from build123d import *

# Parameters (mm, degrees)
SKETCH1_W                 = 60
SKETCH1_H                 = 50
BOSS_EXTRUDE1_DEPTH       = 6.35
CUT_EXTRUDE1_DEPTH        = 6.35
M3_5X0_6_TAPPED_HOLE1_D   = 2.9
M4X0_7_TAPPED_HOLE1_D     = 3.3
M4X0_7_TAPPED_HOLE1_DEPTH = 6.35
M4X0_7_TAPPED_HOLE1_TIP   = 0.991420021


with BuildPart() as part:
    # Sketch1 → Boss-Extrude1 (new body)
    with BuildSketch(Plane(origin=(0, 0, 0), x_dir=(1, 0, 0), z_dir=(0, 1, 0))):
        with Locations((-30, -25)):
            Rectangle(SKETCH1_W, SKETCH1_H)
    extrude(amount=BOSS_EXTRUDE1_DEPTH)

    # Sketch2 → Cut-Extrude1 (cut)
    with BuildSketch(Plane(origin=(0, 6.35, 0), x_dir=(1, 0, 0), z_dir=(0, 1, 0))):
        with BuildLine():
            Line((-26.825, -34.482582718), (-26.825, -20))
            Line((-26.825, -20), (-33.175, -20))
            Line((-33.175, -20), (-33.175, -34.482582718))
            ThreePointArc((-33.175, -34.482582718), (-30, -35), (-26.825, -34.482582718))
        make_face()
        with BuildLine():
            Line((-33.175, -20), (-26.825, -20))
            Line((-26.825, -20), (-26.825, -34.482582718))
            ThreePointArc((-26.825, -34.482582718), (-21.88365846, -30.841660723), (-20, -25))
            ThreePointArc((-20, -25), (-35.841660723, -16.88365846), (-33.175, -34.482582718))
            Line((-33.175, -34.482582718), (-33.175, -20))
        make_face()
        with BuildLine():
            Line((-26.825, -50), (-26.825, -34.482582718))
            ThreePointArc((-26.825, -34.482582718), (-30, -35), (-33.175, -34.482582718))
            Line((-33.175, -34.482582718), (-33.175, -50))
            Line((-33.175, -50), (-26.825, -50))
        make_face()
    extrude(amount=-CUT_EXTRUDE1_DEPTH, mode=Mode.SUBTRACT)

    # M3.5x0.6 Tapped Hole1 (through all)
    with Locations(Plane(origin=(-26.376533369, 6.35, 11.477038432), x_dir=(0, 0, 1), z_dir=(0, 1, 0))):
        with Locations((0, 0), (3.623466631, -13.522961568), (17.146428199, -17.146428199), (23.422456505, 6.276028306)):
            Hole(M3_5X0_6_TAPPED_HOLE1_D / 2)

    # M4x0.7 Tapped Hole1
    with Locations(Plane(origin=(-8, 3.175, 0), x_dir=(-1, 0, 0), z_dir=(0, 0, -1))):
        with Locations((0, 0), (22, 0), (44, 0)):
            Hole(M4X0_7_TAPPED_HOLE1_D / 2, depth=M4X0_7_TAPPED_HOLE1_DEPTH)
            with Locations((0, 0, -(M4X0_7_TAPPED_HOLE1_DEPTH + M4X0_7_TAPPED_HOLE1_TIP / 2))):  # 118° drill point
                Cone(0, M4X0_7_TAPPED_HOLE1_D / 2, M4X0_7_TAPPED_HOLE1_TIP, mode=Mode.SUBTRACT)


solid = part.part
Part model, mm, in its own coordinate system. A direction names the side the tool comes from. Give positions to 0.01 mm unless a question says otherwise; leave off trailing zeros. Order: outer loops, then holes, each group sorted by start corner. A loop starts at its lowest first (then second) coordinate and runs counter-clockwise, first axis right, second up. Notation, with made-up numbers: (10.25, 85) - (19.25, 85) arc R30 ccw to (19.25, 120) - close; hole circle Ø11 at (41, 28.25). An arc over 180 degrees is marked (long way). One line per question, with ' | ' between items.
1. Band-saw the part on B-B on z = 31.5. List the corners of the cut face in (x, y), then the cut area to 3 significant figures.
Filled in:
outline: (-60, 0) - (-37.6, 0) - (-37.6, 6.35) - (-60, 6.35) - close; (-22.4, 0) - (0, 0) - (0, 6.35) - (-22.4, 6.35) - close | area: 284 mm²
2. Drop flat-ended pins along their axis: P1, Ø10, axis at x = -53.5, z = 42.5, coming from the -Y side; P2, Ø3, axis at x = -30, y = 3.175, coming from the +Z side; P3, Ø3, axis at x = -8, y = 3.175, coming from the -Z side. Give the stop position or say it passes through.
Filled in:
P1: y = 0 | P2: z = 15.11 | P3: z = 6.44
3. Drill centre lines: probe 1 along Y at (x, z) = (-30, 4.25) (3 decimals); probe 2 along X at (y, z) = (0.5, 42) (3 decimals); probe 3 along X at (y, z) = (2.5, 3). Where is each one in solid material? Low to high.
Filled in:
probe 1: 0 to 1.525, 4.825 to 6.35 | probe 2: -60 to -33.175, -26.825 to 0 | probe 3: -60 to -53.51, -50.49 to -31.51, -28.49 to -9.51, -6.49 to 0
4. Pull direction X, two halves, no side cores. Call faces 1 (the face through (-60, 3, 25)), 2 (the face through (-8.358, 1.564, 3.219)), 3 (the face through (-14, 3, 50)): +X half, -X half, draft (parallel to the pull), parting line (faces both ways), or undercut.
Filled in:
face 1: -X half | face 2: undercut | face 3: draft
5. Band-saw the part on A-A on z = 42. List the corners of the cut face in (x, y) (3 decimals), then the cut area to 3 significant figures.
Filled in:
outline: (-60, 0) - (-33.175, 0) - (-33.175, 6.35) - (-60, 6.35) - close; (-26.825, 0) - (0, 0) - (0, 6.35) - (-26.825, 6.35) - close | area: 341 mm²
6. Which spindle directions (+Z, -Z, +X, -X, +Y, -Y) get a long thin tool onto all of the face, cutting with end or side? Do faces 4 (the face through (-31.31, 2.17, 3.22)), 5 (the face through (-26.932, 3.131, 10.138)), 6 (the face through (-26.825, 3, 42)). Say none if no direction does.
Filled in:
face 4: -Z | face 5: +Y, -Y | face 6: +Z, +Y, -Y
